Verification items for this drawing (mm, ordinates from the low corner). Round coordinates to 2 decimals unless told otherwise and drop trailing zeros. Order: outer loops, then holes, each group sorted by start corner. A loop starts at its lowest first (then second) coordinate and runs counter-clockwise, first axis right, second up. Notation, with made-up numbers: (-7, 50.5) -> (48, 50.5) arc R26 ccw to (48, 88.5) -> close; hole circle Ø2 at (-26, 60). An arc over 180 degrees is marked (long way). Answer in a Markdown table with one row per item.
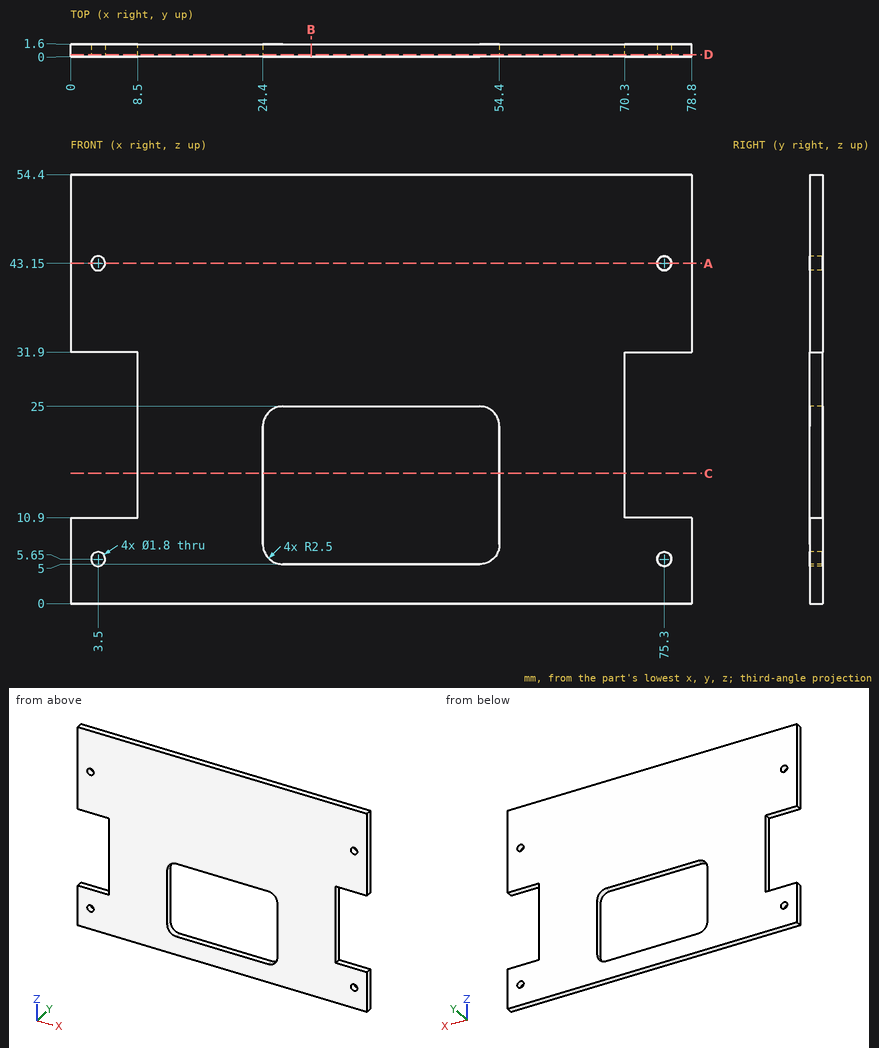
Item 1: Cross-section at B-B (x = 30.5). Record the boundary of the cut face in (y, z).
Result sheet:
| item | result |
|---|---|
| outline | (0, 0) -> (1.6, 0) -> (1.6, 5) -> (0, 5) -> close; (0, 25) -> (1.6, 25) -> (1.6, 54.4) -> (0, 54.4) -> close |
Item 2: Scan lines: line 1 (Z direction, x = 75.3, y = 0.4); line 2 (X direction, y = 1.2, z = 43.15); line 3 (Z direction, x = 35, y = 0.8). Record each from-to range of solid material in increasing order. Write a range as [from, to].
Result sheet:
| item | result |
|---|---|
| line 1 | z = [0, 4.75], [6.55, 10.9], [31.9, 42.25], [44.05, 54.4] |
| line 2 | x = [0, 2.6], [4.4, 74.4], [76.2, 78.8] |
| line 3 | z = [0, 5], [25, 54.4] |
Item 3: Depth check by flat-ended pin: P1, Ø2.5, axis at x = 3.5, z = 5.65, coming from the +Y side; P2, Ø0.8, axis at y = 1, z = 11.5, coming from the +X side; P3, Ø0.8, axis at y = 0.5, z = 15.5, coming from the -X side. Enter the tip coordinate at first touch or a pass-through.
Result sheet:
| item | result |
|---|---|
| P1 | stops at y = 1.6 |
| P2 | stops at x = 70.3 |
| P3 | stops at x = 8.5 |
Item 4: Cross-section at C-C (z = 16.5). Record the boundary of the cut face in (x, y), and give its area (3 significant figures).
Result sheet:
| item | result |
|---|---|
| outline | (8.5, 0) -> (24.4, 0) -> (24.4, 1.6) -> (8.5, 1.6) -> close; (54.4, 0) -> (70.3, 0) -> (70.3, 1.6) -> (54.4, 1.6) -> close |
| area | 50.9 mm^2 |
Item 5: Cross-section at A-A (z = 43.15). Record the boundary of the cut face in (x, y), and give its area (3 significant figures).
Result sheet:
| item | result |
|---|---|
| outline | (0, 0) -> (2.6, 0) -> (2.6, 1.6) -> (0, 1.6) -> close; (4.4, 0) -> (74.4, 0) -> (74.4, 1.6) -> (4.4, 1.6) -> close; (76.2, 0) -> (78.8, 0) -> (78.8, 1.6) -> (76.2, 1.6) -> close |
| area | 120 mm^2 |
Item 6: Cross-section at D-D (y = 0.25). Record the boundary of the cut face in (x, z), and give its area (3 significant figures).
Result sheet:
| item | result |
|---|---|
| outline | (0, 0) -> (78.8, 0) -> (78.8, 10.9) -> (70.3, 10.9) -> (70.3, 31.9) -> (78.8, 31.9) -> (78.8, 54.4) -> (0, 54.4) -> (0, 31.9) -> (8.5, 31.9) -> (8.5, 10.9) -> (0, 10.9) -> close; hole circle Ø1.8 at (3.5, 5.65); hole circle Ø1.8 at (3.5, 43.15); hole (24.4, 7.5) arc R2.5 ccw to (26.9, 5) -> (51.9, 5) arc R2.5 ccw to (54.4, 7.5) -> (54.4, 22.5) arc R2.5 ccw to (51.9, 25) -> (26.9, 25) arc R2.5 ccw to (24.4, 22.5) -> close; hole circle Ø1.8 at (75.3, 5.65); hole circle Ø1.8 at (75.3, 43.15) |
| area | 3,320 mm^2 |
